Source: CAD feature listing. Evaluate the final solid. Frame: model axes, mm. A direction names the side the tool comes from. Coordinates: 2 decimals unless noted, no trailing zeros. Write each loop counter-clockwise with the first axis right and the second up, starting at its lowest first coordinate (ties: lowest second). Pieces come first, ordered by that corner, then holes. Notation, with made-up numbers: (-30.5, 23) -> (0.5, 23) arc R13 ccw to (0.5, 31) -> close; hole circle Ø1 at (74.5, 27). An arc over 180 degrees is marked (long way). One line per item, written item: value. Start each with the question number.
1. Mould query, pull axis X, two halves, no side actions, for faces 1 (the cylindrical face through (18.43, -3.33, 0.6)), 2 (the flat face through (18, -3, 9)), 3 (the cylindrical face through (6.1, -4.2, 1)). Classes: released by +X, released by -X, zero draft, split by the parting line, or undercut.
2. Section query D-D, the plane y = -6. Output: boundary loops of the cut face in (x, z), and give its area (3 significant figures).
3. Section query C-C, the plane y = -4.75. Output: boundary loops of the cut face in (x, z), and give its area (3 significant figures).
4. Section query A-A, the plane z = 5.5. Output: boundary loops of the cut face in (x, y) (3 decimals).
5. Section query B-B, the plane x = 14.5. Output: boundary loops of the cut face in (y, z), and give its area (3 significant figures).
6. Line query: line 1 (Y direction, x = 4.5, z = 1.1); line 2 (X direction, y = -2, z = 0.75); line 3 (X direction, y = -4.75, z = 7.25). Output: solid intervals per line, ascending.
7. First-contact query: P1, Ø2, axis at y = -3, z = 4, coming from the -X side; P2, Ø3.5, axis at y = -3.375, z = 5.5, coming from the +X side. Flat tips, straight axial feed; report the tip coordinate or a pass-through.
8. Access query for faces 4 (the flat face through (9, -3, 2)), 5 (the flat face through (11.6, 0, 1.8)). Directions: +Z, -Z, +X, -X, +Y, -Y. A direction counts if a zero-diameter tool reaches every point of the face in a straight line with its end or side. Return the directions, or none.
from build123d import *

# Parameters (mm, degrees)
ESQUISSE1_W             = 19
ESQUISSE1_H             = 6.75
BOSS_EXTRU_1_DEPTH      = 2
ESQUISSE4_R             = 2
ENL_V_MAT_EXTRU_1_DEPTH = 10
ESQUISSE6_W             = 1.5
ESQUISSE6_H             = 6.75
BOSS_EXTRU_2_DEPTH      = 7
CONG_1_R                = 2
ESQUISSE7_R             = 2.1
ENL_V_MAT_EXTRU_2_DEPTH = 3


with BuildPart() as part:
    # Esquisse1 → Boss.-Extru.1 (new body)
    with BuildSketch(Plane.XY):
        with Locations((9.5, -3.375)):
            Rectangle(ESQUISSE1_W, ESQUISSE1_H)
    extrude(amount=BOSS_EXTRU_1_DEPTH)

    # Esquisse4 → Enlèv. mat.-Extru.1 (cut)
    with BuildSketch(Plane(origin=(0, 0, 0), x_dir=(-1, 0, 0), z_dir=(0, 0, -1))):
        with Locations((-14.5, -3)):
            Circle(ESQUISSE4_R)
        with Locations((-4.5, -3)):
            Circle(ESQUISSE4_R)
    extrude(amount=-ENL_V_MAT_EXTRU_1_DEPTH, mode=Mode.SUBTRACT)

    # Esquisse6 → Boss.-Extru.2 (add)
    with BuildSketch(Plane.XY.offset(2)):
        with Locations((18.25, -3.375)):
            Rectangle(ESQUISSE6_W, ESQUISSE6_H)
    extrude(amount=BOSS_EXTRU_2_DEPTH)

    # Congé1
    cong_1_edges = [part.edges().sort_by_distance(p)[0] for p in [
        (19, -3.375, 0),
    ]]
    fillet(cong_1_edges, radius=CONG_1_R)

    # Esquisse7 → Enlèv. mat.-Extru.2 (cut)
    with BuildSketch(Plane.ZY.offset(-17.5)):
        with Locations((5.5, -3.375)):
            Circle(ESQUISSE7_R)
    extrude(amount=-ENL_V_MAT_EXTRU_2_DEPTH, mode=Mode.SUBTRACT)


solid = part.part
Computed values:
1. face 1: released by +X
1. face 2: zero draft
1. face 3: undercut
2. outline: (0, 0) -> (17, 0) arc R2 ccw to (19, 2) -> (19, 9) -> (17.5, 9) -> (17.5, 2) -> (0, 2) -> close
2. area: 47.6 mm²
3. outline: (0, 0) -> (3.53, 0) -> (3.53, 2) -> (0, 2) -> close; (5.47, 0) -> (13.53, 0) -> (13.53, 2) -> (5.47, 2) -> close; (15.47, 0) -> (17, 0) arc R2 ccw to (19, 2) -> (19, 3.91) -> (17.5, 3.91) -> (17.5, 2) -> (15.47, 2) -> close; (17.5, 7.09) -> (19, 7.09) -> (19, 9) -> (17.5, 9) -> close
3. area: 35.1 mm²
4. outline: (17.5, -6.75) -> (19, -6.75) -> (19, -5.475) -> (17.5, -5.475) -> close; (17.5, -1.275) -> (19, -1.275) -> (19, 0) -> (17.5, 0) -> close
5. outline: (-6.75, 0) -> (-5, 0) -> (-5, 2) -> (-6.75, 2) -> close; (-1, 0) -> (0, 0) -> (0, 2) -> (-1, 2) -> close
5. area: 5.50 mm²
6. line 1: y = -6.75 to -5, -1 to 0
6. line 2: x = 0 to 2.77, 6.23 to 12.77, 16.23 to 18.56
6. line 3: x = 17.5 to 19
7. P1: stops at x = 17.5
7. P2: passes through
8. face 4: +Z, -X, +Y, -Y
8. face 5: +Z, -Z, +X, -X, +Y
